Model file for the job. Use its own axes, mm. A direction names the side the tool comes from. Give positions to 0.01 mm unless a question says otherwise; leave off trailing zeros. Write each loop counter-clockwise with the first axis right and the second up, starting at its lowest first coordinate (ties: lowest second). Pieces come first, ordered by that corner, then holes. Notation, with made-up numbers: (58.5, 42) - (69.5, 42) arc R28 cw to (69.5, 73) - close; hole circle Ø6 at (30, -33). An arc over 180 degrees is marked (long way). One line per item, written item: value. Start each with the question number.
(1) Probe L1, parallel to X at y = 1.45, z = -38.5; L2, parallel to X at y = 0.65, z = -21.5; L3, parallel to X at y = 2.5, z = -10. List the from-to ranges inside material, lowest first.
(2) 3-axis set-ups, long thin cutter, end or side, ignore diameter. For faces 4 (the face through (-23, 8, -3)), 5 (the face through (-23, 0, -3)), 6 (the face through (-40, 1, -20)): which of +Z, -Z, +X, -X, +Y, -Y reach the whole face in a straight line?
(3) Cut at A-A, the plane z = -21.5. List the corners of the cut face in (x, y), and give its area (3 significant figures).
(4) Mould opens along Z. For faces 1 (the face through (-22, 1, -40)), 2 (the face through (-23.237, 7.176, -1.479)), 3 (the face through (-5, 1, -20)) say: pulls with the +Z half, pulls with the -Z half, needs draft (parallel to the pull), parting line crosses it, or undercut.
(5) Cut at B-B, the plane x = -43.5. List the corners of the cut face in (y, z), and give its area (3 significant figures).
(6) Cut at D-D, the plane x = -8. List the corners of the cut face in (y, z), and give its area (3 significant figures).
(7) Cut at C-C, the plane z = -38.5. List the corners of the cut face in (x, y).
(8) Drop flat-ended pins along their axis: P1, Ø2.5, axis at x = -1.5, z = -38.5, coming from the +Y side; P2, Ø1.8, axis at x = -43.5, z = -38.5, coming from the +Y side; P3, Ø1.5, axis at x = -18, y = 4.5, coming from the -Z side. Give the stop position or say it passes through.
from build123d import *

# Parameters (mm, degrees)
SKETCH2_W                 = 5
SKETCH2_H                 = 40
SKETCH2_W_2               = 35
SKETCH2_H_2               = 5
BOSS_EXTRUDE1_DEPTH       = 3
F_2_0MM_DOWEL_HOLE1_D     = 2
F_2_0MM_DOWEL_HOLE1_DEPTH = 12.029
F_2_0MM_DOWEL_HOLE1_TIP   = 0.600860619
SKETCH4_W                 = 45
SKETCH4_H                 = 3
BOSS_EXTRUDE2_DEPTH       = 10
F_2_0MM_DOWEL_HOLE2_D     = 2
F_2_0MM_DOWEL_HOLE2_DEPTH = 12
F_2_0MM_DOWEL_HOLE2_TIP   = 0.600860619


with BuildPart() as part:
    # Sketch2 → Boss-Extrude1 (new body)
    with BuildSketch(Plane(origin=(0, 0, 0), x_dir=(1, 0, 0), z_dir=(0, 1, 0))):
        with Locations((-42.5, 20)):
            Rectangle(SKETCH2_W, SKETCH2_H)
        with Locations((-22.5, 37.5)):
            Rectangle(SKETCH2_W_2, SKETCH2_H_2)
        with Locations((-2.5, 20)):
            Rectangle(SKETCH2_W, SKETCH2_H)
        with Locations((-22.5, 2.5)):
            Rectangle(SKETCH2_W_2, SKETCH2_H_2)
    extrude(amount=BOSS_EXTRUDE1_DEPTH)

    # Ø2.0mm Dowel Hole1
    with Locations(Plane(origin=(-1.5, 0, -38.5), x_dir=(0, 0, -1), z_dir=(0, -1, 0))):
        with Locations((0, 0), (0, -42), (-17, 0), (-17, -42)):
            Hole(F_2_0MM_DOWEL_HOLE1_D / 2, depth=F_2_0MM_DOWEL_HOLE1_DEPTH)
            with Locations((0, 0, -(F_2_0MM_DOWEL_HOLE1_DEPTH + F_2_0MM_DOWEL_HOLE1_TIP / 2))):  # 118° drill point
                Cone(0, F_2_0MM_DOWEL_HOLE1_D / 2, F_2_0MM_DOWEL_HOLE1_TIP, mode=Mode.SUBTRACT)

    # Sketch4 → Boss-Extrude2 (add)
    with BuildSketch(Plane(origin=(0, 3, 0), x_dir=(1, 0, 0), z_dir=(0, 1, 0))):
        with Locations((-22.5, 1.5)):
            Rectangle(SKETCH4_W, SKETCH4_H)
    extrude(amount=BOSS_EXTRUDE2_DEPTH)

    # Ø2.0mm Dowel Hole2
    with Locations(Plane(origin=(0, 0, -3), x_dir=(-1, 0, 0), z_dir=(0, 0, -1))):
        with Locations((22.5, 6.5)):
            Hole(F_2_0MM_DOWEL_HOLE2_D / 2, depth=F_2_0MM_DOWEL_HOLE2_DEPTH)
            with Locations((0, 0, -(F_2_0MM_DOWEL_HOLE2_DEPTH + F_2_0MM_DOWEL_HOLE2_TIP / 2))):  # 118° drill point
                Cone(0, F_2_0MM_DOWEL_HOLE2_D / 2, F_2_0MM_DOWEL_HOLE2_TIP, mode=Mode.SUBTRACT)


solid = part.part
Answers follow:
1. L1: x = -45 to -44.5, -42.5 to -2.5, -0.5 to 0
1. L2: x = -45 to -44.5, -42.5 to -40, -5 to -2.5, -0.5 to 0
1. L3: x = -45 to -40, -5 to 0
2. face 4: -Z, +X, -X, +Y
2. face 5: +Z, -Z, +X, -X, -Y
2. face 6: +Y, -Y
3. outline: (-45, 0) - (-44.5, 0) - (-44.5, 3) - (-45, 3) - close; (-42.5, 0) - (-40, 0) - (-40, 3) - (-42.5, 3) - close; (-5, 0) - (-2.5, 0) - (-2.5, 3) - (-5, 3) - close; (-0.5, 0) - (0, 0) - (0, 3) - (-0.5, 3) - close
3. area: 18.0 mm²
4. face 1: pulls with the -Z half
4. face 2: needs draft
4. face 3: undercut
5. outline: (0, -40) - (3, -40) - (3, -39.5) - (0, -39.5) - close; (0, -37.5) - (3, -37.5) - (3, -22.5) - (0, -22.5) - close; (0, -20.5) - (3, -20.5) - (3, -3) - (13, -3) - (13, 0) - (0, 0) - close
5. area: 138 mm²
6. outline: (0, -40) - (3, -40) - (3, -35) - (0, -35) - close; (0, -5) - (3, -5) - (3, -3) - (13, -3) - (13, 0) - (0, 0) - close
6. area: 60.0 mm²
7. outline: (-45, 0) - (-44.5, 0) - (-44.5, 3) - (-45, 3) - close; (-42.5, 0) - (-2.5, 0) - (-2.5, 3) - (-42.5, 3) - close; (-0.5, 0) - (0, 0) - (0, 3) - (-0.5, 3) - close
8. P1: stops at y = 3
8. P2: passes through
8. P3: stops at z = -3
